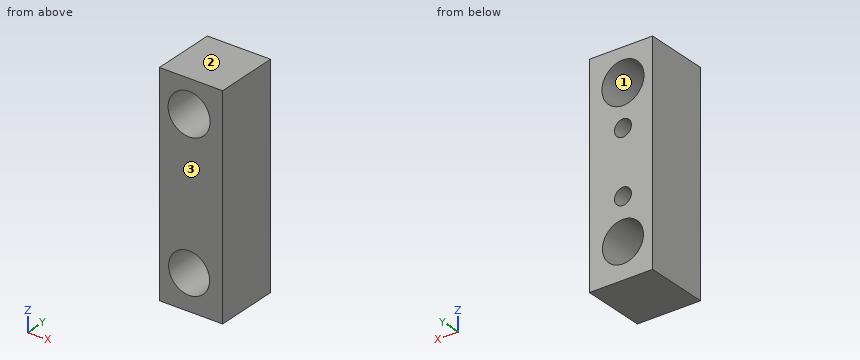
```python
from build123d import *

# Parameters (mm, degrees)
SKETCH1_W           = 203.448651213
SKETCH1_H           = 60.760194486
BOSS_EXTRUDE1_DEPTH = 60
SKETCH2_R           = 19.434497102
SKETCH2_R_2         = 19.923805808
CUT_EXTRUDE2_DEPTH  = 80
SKETCH3_R           = 8
CUT_EXTRUDE3_DEPTH  = 45


with BuildPart() as part:
    # Sketch1 → Boss-Extrude1 (new body)
    with BuildSketch(Plane(origin=(0, 0, 0), x_dir=(0, 0, -1), z_dir=(1, 0, 0))):
        with Locations((-0.196000627, -1.960006274)):
            Rectangle(SKETCH1_W, SKETCH1_H)
    extrude(amount=BOSS_EXTRUDE1_DEPTH)

    # Sketch2 → Cut-Extrude2 (cut)
    with BuildSketch(Plane(origin=(0, 28.420090969, 0), x_dir=(-1, 0, 0), z_dir=(0, 1, 0))):
        with Locations(Location((-28.157475654, -67.835345713, 0), (0, 0, 90))):  # turned: the seam where the file's is
            Circle(SKETCH2_R)
        with Locations(Location((-28.157475654, 70.713811049, 0), (0, 0, 90))):  # turned: the seam where the file's is
            Circle(SKETCH2_R_2)
    extrude(amount=-CUT_EXTRUDE2_DEPTH, mode=Mode.SUBTRACT)

    # Sketch3 → Cut-Extrude3 (cut)
    with BuildSketch(Plane(origin=(0, 28.420090969, 0), x_dir=(1, 0, 0), z_dir=(0, 1, 0))):
        with Locations(Location((28.157475654, 28.339432247, 0), (0, 0, 270))):  # turned: the seam where the file's is
            Circle(SKETCH3_R)
        with Locations(Location((28.157475654, -31.26607036, 0), (0, 0, 270))):  # turned: the seam where the file's is
            Circle(SKETCH3_R)
    extrude(amount=-CUT_EXTRUDE3_DEPTH, mode=Mode.SUBTRACT)


solid = part.part
```
Geometry: final body of the model. Coordinates: model frame, mm. Face numbers are marked on the shaded views. Coordinates: 2 decimals unless noted, no trailing zeros. Loops run counter-clockwise (first coordinate to the right, second up) from the corner with the lowest first, then second, coordinate; pieces in that order, holes last. Notation, with made-up numbers: (46.25, 22.25) -> (79.25, 22.25) arc R16 ccw to (79.25, 50.25) -> close; hole circle Ø10 at (-37.5, 52). An arc over 180 degrees is marked (long way). Use a Markdown table: item, result. Add a question column.
(1) Line query: line 1 along Z through (x, y) = (42, 15); line 2 along Z through (x, y) = (13.5, -1); line 3 along X through (y, z) = (-23, 72). Output: solid intervals per line, ascending.
(2) Mould query, pull axis Z, two halves, no side actions, for the marked faces 1, 2 and 3. Classes: pulls with the +Z half, pulls with the -Z half, needs draft (parallel to the pull), parting line crosses it, or undercut.
(3) Section query B-B, the plane x = 17.5. Return loops of the section in (y, z), plus the area to 3 significant figures.
(4) Section query A-A, the plane z = -72. Return loops of the section in (x, y), plus the area to 3 significant figures.
(5) Section query D-D, the plane z = -25. Return loops of the section in (x, y), plus the area to 3 significant figures.
(6) Section query C-C, the plane y = -10.5. Return loops of the section in (x, z), plus the area to 3 significant figures.
Answer:
| question | item | result |
|---|---|---|
| 1 | line 1 | z = -101.53 to -81.48, -54.19 to 56.38, 85.04 to 101.92 |
| 1 | line 2 | z = -101.53 to -80.6, -55.07 to 57.22, 84.21 to 101.92 |
| 1 | line 3 | x = 0 to 8.28, 48.04 to 60 |
| 2 | face 1 | undercut |
| 2 | face 2 | pulls with the +Z half |
| 2 | face 3 | needs draft |
| 3 | outline | (-32.34, -101.53) -> (28.42, -101.53) -> (28.42, -84.09) -> (-32.34, -84.09) -> close; (-32.34, -51.58) -> (28.42, -51.58) -> (28.42, 53.88) -> (-32.34, 53.88) -> close; (-32.34, 87.55) -> (28.42, 87.55) -> (28.42, 101.92) -> (-32.34, 101.92) -> close |
| 3 | area | 8,340 mm^2 |
| 4 | outline | (0, -32.34) -> (9.17, -32.34) -> (9.17, 28.42) -> (0, 28.42) -> close; (47.14, -32.34) -> (60, -32.34) -> (60, 28.42) -> (47.14, 28.42) -> close |
| 4 | area | 1,340 mm^2 |
| 5 | outline | (0, -32.34) -> (60, -32.34) -> (60, 28.42) -> (35.43, 28.42) -> (35.43, -16.58) -> (20.89, -16.58) -> (20.89, 28.42) -> (0, 28.42) -> close |
| 5 | area | 2,990 mm^2 |
| 6 | outline | (0, -101.53) -> (60, -101.53) -> (60, 101.92) -> (0, 101.92) -> close; hole circle Ø39.85 at (28.16, 70.71); hole circle Ø38.87 at (28.16, -67.84); hole circle Ø16 at (28.16, -28.34); hole circle Ø16 at (28.16, 31.27) |
| 6 | area | 9,370 mm^2 |
